Verification items for the finished model (mm, model axes). Face numbers are marked on the shaded views. A direction names the side the tool comes from. Round coordinates to 2 decimals unless told otherwise and drop trailing zeros. Write each loop counter-clockwise with the first axis right and the second up, starting at its lowest first coordinate (ties: lowest second). Pieces come first, ordered by that corner, then holes.
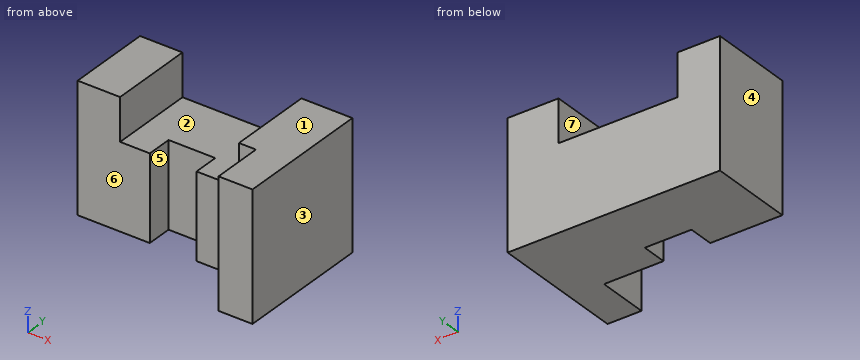
from build123d import *

# Parameters (mm, degrees)
F0_W     = 17.5
F0_H     = 50
F1_DEPTH = 50
F2_W     = 35
F2_H     = 50
F3_DEPTH = 27.5
F4_W     = 50
F4_H     = 50
F5_DEPTH = 25
F6_W     = 50
F6_H     = 75
F7_DEPTH = 30
F8_W     = 20
F8_H     = 75
F9_DEPTH = 30


with BuildPart() as f1:
    # F0 (on Front) → F1 (new body)
    with BuildSketch(Plane.XZ):
        Polygon((0, 75), (0, 0), (25, 0), (25, 50), (25, 75), align=None)
        with Locations((33.75, 25)):
            Rectangle(F0_W, F0_H)
    extrude(amount=F1_DEPTH)

    # F2 (on face) → F3 (join)
    with BuildSketch(Plane.YZ.offset(42.5)):
        with Locations((-17.5, 25)):
            Rectangle(F2_W, F2_H)
    extrude(amount=F3_DEPTH)

    # F4 (on face) → F5 (join)
    with BuildSketch(Plane.YZ.offset(70)):
        with Locations((-25, 25)):
            Rectangle(F4_W, F4_H)
    extrude(amount=F5_DEPTH)

    # F6 (on face) → F7 (join)
    with BuildSketch(Plane.YZ.offset(95)):
        with Locations((-25, 37.5)):
            Rectangle(F6_W, F6_H)
    extrude(amount=F7_DEPTH)

    # F8 (on face) → F9 (join)
    with BuildSketch(Plane.XZ.offset(50)):
        with Locations((115, 37.5)):
            Rectangle(F8_W, F8_H)
    extrude(amount=F9_DEPTH)


solid = f1.part
Q1. Depth check by flat-ended pin: P1, Ø13, axis at x = 28.5, z = 29.5, coming from the -Y side; P2, Ø24, axis at y = -70.5, z = 45.5, coming from the -X side. Enter the tip coordinate at first touch or a pass-through.
Recorded:
P1: stops at y = -50
P2: stops at x = 105
Q2. Material ranges on line 1 along X through (y, z) = (-42, 19.5); line 2 along X through (y, z) = (-6, 56.5); line 3 along Y through (x, z) = (95, 34), recorded low to high.
Recorded:
line 1: x = 0 to 42.5, 70 to 125
line 2: x = 0 to 25, 95 to 125
line 3: y = -50 to 0
Q3. Release check for a two-part mould opening along X. For the marked faces 1, 2, 3 and 4 record: released by +X, released by -X, zero draft, split by the parting line, or undercut.
Recorded:
face 1: zero draft
face 2: undercut
face 3: released by +X
face 4: released by -X
Q4. Sectioned sample at D-D (z = 19). Enter the section's corners in (x, y).
Recorded:
outline: (0, -50) - (42.5, -50) - (42.5, -35) - (70, -35) - (70, -50) - (105, -50) - (105, -80) - (125, -80) - (125, 0) - (0, 0) - close
Q5. Sectioned sample at A-A (z = 62). Enter the section's corners in (x, y), plus the area to 3 significant figures.
Recorded:
outline: (0, -50) - (25, -50) - (25, 0) - (0, 0) - close; (95, -50) - (105, -50) - (105, -80) - (125, -80) - (125, 0) - (95, 0) - close
area: 3,350 mm2
Q6. Tool access check on the marked faces 5, 6 and 7. Record the directions out of +Z, -Z, +X, -X, +Y, -Y that give a thin tool (end or side, any length) a straight path to the whole face; none if there is none.
Recorded:
face 5: +Z, -Z, -Y
face 6: +Z, -Z, -X, -Y
face 7: +Z, +Y, -Y
Q7. Sectioned sample at B-B (y = -45). Enter the section's corners in (x, z).
Recorded:
outline: (0, 0) - (42.5, 0) - (42.5, 50) - (25, 50) - (25, 75) - (0, 75) - close; (70, 0) - (125, 0) - (125, 75) - (95, 75) - (95, 50) - (70, 50) - close
Q8. Sectioned sample at C-C (y = -17.5). Enter the section's corners in (x, z), plus the area to 4 significant figures.
Recorded:
outline: (0, 0) - (125, 0) - (125, 75) - (95, 75) - (95, 50) - (25, 50) - (25, 75) - (0, 75) - close
area: 7,625 mm2
